from build123d import *

# Parameters (mm, degrees)
F0_W     = 1.2
F0_H     = 1.2
F0_W_2   = 2.6
F0_H_2   = 107.6
F1_DEPTH = 0.7
F2_DEPTH = 25
F2_TAPER = 3
F3_DEPTH = 25
F3_TAPER = 3
F5_DEPTH = 0.7
F7_DEPTH = 0.7
F8_R     = 1.4


with BuildPart() as f1:
    # F0 (on Top) → F1 (new body)
    with BuildSketch(Plane.XY):
        with BuildLine():
            Line((-2.5, 55), (-39.2, 55))
            ThreePointArc((-39.2, 55), (-50.3722871427, 50.3722871427), (-55, 39.2))
            Line((-55, 39.2), (-55, -39.2))
            ThreePointArc((-55, -39.2), (-50.3722871427, -50.3722871427), (-39.2, -55))
            Line((-39.2, -55), (-2.5, -55))
            Line((-2.5, -55), (-2.5, -53.8))
            Line((-2.5, -53.8), (-38.8, -53.8))
            ThreePointArc((-38.8, -53.8), (-49.4066017178, -49.4066017178), (-53.8, -38.8))
            Line((-53.8, -38.8), (-53.8, 38.8))
            ThreePointArc((-53.8, 38.8), (-49.4066017178, 49.4066017178), (-38.8, 53.8))
            Line((-38.8, 53.8), (-2.5, 53.8))
            Line((-2.5, 53.8), (-2.5, 55))
        make_face()
        with Locations((-1.9, 54.4)):
            Rectangle(F0_W, F0_H)
        with Locations((0, 54.4)):
            Rectangle(F0_W_2, F0_H)
        with Locations((1.9, 54.4)):
            Rectangle(F0_W, F0_H)
        with BuildLine():
            Line((39.2, 55), (2.5, 55))
            Line((2.5, 55), (2.5, 53.8))
            Line((2.5, 53.8), (38.8, 53.8))
            ThreePointArc((38.8, 53.8), (49.4066017178, 49.4066017178), (53.8, 38.8))
            Line((53.8, 38.8), (53.8, -38.8))
            ThreePointArc((53.8, -38.8), (49.4066017178, -49.4066017178), (38.8, -53.8))
            Line((38.8, -53.8), (2.5, -53.8))
            Line((2.5, -53.8), (2.5, -55))
            Line((2.5, -55), (39.2, -55))
            ThreePointArc((39.2, -55), (50.3722871427, -50.3722871427), (55, -39.2))
            Line((55, -39.2), (55, 39.2))
            ThreePointArc((55, 39.2), (50.3722871427, 50.3722871427), (39.2, 55))
        make_face()
        with Locations((-1.9, -54.4)):
            Rectangle(F0_W, F0_H)
        with Locations((-1.9, 0)):
            Rectangle(F0_W, F0_H_2)
        with Locations((1.9, 0)):
            Rectangle(F0_W, F0_H_2)
        with Locations((0, -54.4)):
            Rectangle(F0_W_2, F0_H)
        Rectangle(F0_W_2, F0_H_2)
        with Locations((1.9, -54.4)):
            Rectangle(F0_W, F0_H)
    extrude(amount=F1_DEPTH)

    # F0 (on Top) → F2 (join)
    with BuildSketch(Plane.XY):
        with Locations((1.9, 54.4)):
            Rectangle(F0_W, F0_H)
        with Locations((1.9, -54.4)):
            Rectangle(F0_W, F0_H)
        with Locations((1.9, 0)):
            Rectangle(F0_W, F0_H_2)
        with BuildLine():
            Line((39.2, 55), (2.5, 55))
            Line((2.5, 55), (2.5, 53.8))
            Line((2.5, 53.8), (38.8, 53.8))
            ThreePointArc((38.8, 53.8), (49.4066017178, 49.4066017178), (53.8, 38.8))
            Line((53.8, 38.8), (53.8, -38.8))
            ThreePointArc((53.8, -38.8), (49.4066017178, -49.4066017178), (38.8, -53.8))
            Line((38.8, -53.8), (2.5, -53.8))
            Line((2.5, -53.8), (2.5, -55))
            Line((2.5, -55), (39.2, -55))
            ThreePointArc((39.2, -55), (50.3722871427, -50.3722871427), (55, -39.2))
            Line((55, -39.2), (55, 39.2))
            ThreePointArc((55, 39.2), (50.3722871427, 50.3722871427), (39.2, 55))
        make_face()
        with BuildLine():
            Line((38.8, 53.8), (2.5, 53.8))
            Line((2.5, 53.8), (2.5, -53.8))
            Line((2.5, -53.8), (38.8, -53.8))
            ThreePointArc((38.8, -53.8), (49.4066017178, -49.4066017178), (53.8, -38.8))
            Line((53.8, -38.8), (53.8, 38.8))
            ThreePointArc((53.8, 38.8), (49.4066017178, 49.4066017178), (38.8, 53.8))
        make_face()
        with Locations((-1.9, 0)):
            Rectangle(F0_W, F0_H_2)
        with Locations((-1.9, -54.4)):
            Rectangle(F0_W, F0_H)
        with BuildLine():
            Line((-2.5, 55), (-39.2, 55))
            ThreePointArc((-39.2, 55), (-50.3722871427, 50.3722871427), (-55, 39.2))
            Line((-55, 39.2), (-55, -39.2))
            ThreePointArc((-55, -39.2), (-50.3722871427, -50.3722871427), (-39.2, -55))
            Line((-39.2, -55), (-2.5, -55))
            Line((-2.5, -55), (-2.5, -53.8))
            Line((-2.5, -53.8), (-38.8, -53.8))
            ThreePointArc((-38.8, -53.8), (-49.4066017178, -49.4066017178), (-53.8, -38.8))
            Line((-53.8, -38.8), (-53.8, 38.8))
            ThreePointArc((-53.8, 38.8), (-49.4066017178, 49.4066017178), (-38.8, 53.8))
            Line((-38.8, 53.8), (-2.5, 53.8))
            Line((-2.5, 53.8), (-2.5, 55))
        make_face()
        with Locations((-1.9, 54.4)):
            Rectangle(F0_W, F0_H)
        with BuildLine():
            Line((-2.5, -53.8), (-2.5, 53.8))
            Line((-2.5, 53.8), (-38.8, 53.8))
            ThreePointArc((-38.8, 53.8), (-49.4066017178, 49.4066017178), (-53.8, 38.8))
            Line((-53.8, 38.8), (-53.8, -38.8))
            ThreePointArc((-53.8, -38.8), (-49.4066017178, -49.4066017178), (-38.8, -53.8))
            Line((-38.8, -53.8), (-2.5, -53.8))
        make_face()
    extrude(amount=F2_DEPTH, taper=F2_TAPER)

    # F0 (on Top) → F3 (cut)
    with BuildSketch(Plane.XY):
        with BuildLine():
            Line((-2.5, -53.8), (-2.5, 53.8))
            Line((-2.5, 53.8), (-38.8, 53.8))
            ThreePointArc((-38.8, 53.8), (-49.4066017178, 49.4066017178), (-53.8, 38.8))
            Line((-53.8, 38.8), (-53.8, -38.8))
            ThreePointArc((-53.8, -38.8), (-49.4066017178, -49.4066017178), (-38.8, -53.8))
            Line((-38.8, -53.8), (-2.5, -53.8))
        make_face()
        with BuildLine():
            Line((38.8, 53.8), (2.5, 53.8))
            Line((2.5, 53.8), (2.5, -53.8))
            Line((2.5, -53.8), (38.8, -53.8))
            ThreePointArc((38.8, -53.8), (49.4066017178, -49.4066017178), (53.8, -38.8))
            Line((53.8, -38.8), (53.8, 38.8))
            ThreePointArc((53.8, 38.8), (49.4066017178, 49.4066017178), (38.8, 53.8))
        make_face()
    extrude(amount=F3_DEPTH, taper=F3_TAPER, mode=Mode.SUBTRACT)

    # F4 (on face) → F5 (join)
    with BuildSketch(Plane.XY.offset(25)):
        with BuildLine():
            Line((39.2, 53.6898055179), (2.6101944821, 53.6898055179))
            Line((2.6101944821, 53.6898055179), (2.6101944821, -53.6898055179))
            Line((2.6101944821, -53.6898055179), (39.2, -53.6898055179))
            ThreePointArc((39.2, -53.6898055179), (49.4458397398, -49.4458397398), (53.6898055179, -39.2))
            Line((53.6898055179, -39.2), (53.6898055179, 39.2))
            ThreePointArc((53.6898055179, 39.2), (49.4458397398, 49.4458397398), (39.2, 53.6898055179))
        make_face()
    extrude(amount=F5_DEPTH)

    # F6 (on face) → F7 (join)
    with BuildSketch(Plane.XY.offset(25)):
        with BuildLine():
            Line((-39.2, -53.6898055179), (-2.6101944821, -53.6898055179))
            Line((-2.6101944821, -53.6898055179), (-2.6101944821, 53.6898055179))
            Line((-2.6101944821, 53.6898055179), (-39.2, 53.6898055179))
            ThreePointArc((-39.2, 53.6898055179), (-49.4458397398, 49.4458397398), (-53.6898055179, 39.2))
            Line((-53.6898055179, 39.2), (-53.6898055179, -39.2))
            ThreePointArc((-53.6898055179, -39.2), (-49.4458397398, -49.4458397398), (-39.2, -53.6898055179))
        make_face()
    extrude(amount=F7_DEPTH)

    # F8
    f8_edges = [f1.edges().sort_by_distance(p)[0] for p in [
        (1.336685, 0, 0.7),
        (-1.336685, 0, 0.7),
    ]]
    fillet(f8_edges, radius=F8_R)


solid = f1.part
CAD build for the part. Positions are in the model's coordinates, mm. A direction names the side the tool comes from. Give positions to 0.01 mm unless a question says otherwise; leave off trailing zeros. Loops run counter-clockwise (first coordinate to the right, second up) from the corner with the lowest first, then second, coordinate; pieces in that order, holes last. Notation, with made-up numbers: M 2,81 L 7,81 A25 cw 7,113 Z; hole C -19,14.5 d10. An arc over 180 degrees is marked long. Answer in a Markdown table with one row per item. Add a question column.
Item 1: Drop flat-ended pins along their axis: P1, Ø3, axis at y = -12, z = 8.5, coming from the -X side; P2, Ø6, axis at y = -17, z = 12, coming from the -X side; P3, Ø0.8, axis at x = -25.5, z = 25.5, coming from the -Y side; P4, Ø12, axis at y = -43.5, z = 4, coming from the +X side. Give the stop position or say it passes through.
Item 2: Probe probe 1 along X at (y, z) = (-25, 2); probe 2 along X at (y, z) = (-33.5, 18); probe 3 along Y at (x, z) = (-13.5, 5.75). List the from-to ranges inside material, lowest first.
Item 3: Mould opens along X. For faces 1 (the face through (-53.154, -0.543, 12.325)), 2 (the face through (-49.33, 49.56, 25.35)), 3 (the face through (49.33, -49.56, 25.35)), 4 (the face through (19.33, 54.335, 12.68)) say: +X half, -X half, draft (parallel to the pull), parting line (faces both ways), or undercut.
Item 4: Band-saw the part on D-D on z = 20. Give the cut face in (x, y).
Item 5: Band-saw the part on A-A on z = 12.5. Give the cut face in (x, y), then the cut area to 3 significant figures.
Item 6: Tool access for faces 5 (the face through (-28, 1, 25)), 6 (the face through (50.249, -50.494, 0.345)), 7 (the face through (-2, 0.77, 13.35)): list every direction of +Z, -Z, +X, -X, +Y, -Y with a clear straight run to the whole face (end or side of a thin tool).
Reply:
| question | item | result |
|---|---|---|
| 1 | P1 | stops at x = -54.63 |
| 1 | P2 | stops at x = -54.53 |
| 1 | P3 | stops at y = -53.69 |
| 1 | P4 | stops at x = 55 |
| 2 | probe 1 | x = -54.9 to -53.7, -2.6 to -1.4, 1.4 to 2.6, 53.7 to 54.9 |
| 2 | probe 2 | x = -54.06 to -52.86, -3.44 to -2.24, 2.24 to 3.44, 52.86 to 54.06 |
| 2 | probe 3 | y = -54.7 to -53.5, 53.5 to 54.7 |
| 3 | face 1 | undercut |
| 3 | face 2 | -X half |
| 3 | face 3 | +X half |
| 3 | face 4 | draft |
| 4 | outline | M -53.95,-39.2 A14.75 ccw -39.2,-53.95 L -2.35,-53.95 L -2.35,53.95 L -39.2,53.95 A14.75 ccw -53.95,39.2 Z; M 2.35,-53.95 L 39.2,-53.95 A14.75 ccw 53.95,-39.2 L 53.95,39.2 A14.75 ccw 39.2,53.95 L 2.35,53.95 Z; hole M -52.75,-38.8 A13.95 ccw -38.8,-52.75 L -3.55,-52.75 L -3.55,52.75 L -38.8,52.75 A13.95 ccw -52.75,38.8 Z; hole M 3.55,-52.75 L 38.8,-52.75 A13.95 ccw 52.75,-38.8 L 52.75,38.8 A13.95 ccw 38.8,52.75 L 3.55,52.75 Z |
| 5 | outline | M -54.34,-39.2 A15.14 ccw -39.2,-54.34 L -1.96,-54.34 L -1.96,54.34 L -39.2,54.34 A15.14 ccw -54.34,39.2 Z; M 1.96,-54.34 L 39.2,-54.34 A15.14 ccw 54.34,-39.2 L 54.34,39.2 A15.14 ccw 39.2,54.34 L 1.96,54.34 Z; hole M -53.14,-38.8 A14.34 ccw -38.8,-53.14 L -3.16,-53.14 L -3.16,53.14 L -38.8,53.14 A14.34 ccw -53.14,38.8 Z; hole M 3.16,-53.14 L 38.8,-53.14 A14.34 ccw 53.14,-38.8 L 53.14,38.8 A14.34 ccw 38.8,53.14 L 3.16,53.14 Z |
| 5 | area | 741 mm^2 |
| 6 | face 5 | -Z |
| 6 | face 6 | +Z, -Z, +X, -Y |
| 6 | face 7 | +Z, +Y, -Y |
